The drawing under review shows one solid part. Ordinate dimensions are in mm from its lowest x, y, z. Give positions to 0.01 mm unless a question says otherwise; leave off trailing zeros. Order: outer loops, then holes, each group sorted by start corner. A loop starts at its lowest first (then second) coordinate and runs counter-clockwise, first axis right, second up. Notation, with made-up numbers: (27.25, -36) - (66.25, -36) arc R16 ccw to (66.25, -30) - close; hole circle Ø2 at (42.25, -2). An arc over 180 degrees is marked (long way). Use CSV: the item, a comma, the result in double quotes. Start each with the question number.
1. To check wall thickness, follow line 1 (Y direction, x = 57.15, z = 5); line 2 (Y direction, x = 58, z = 7.75); line 3 (X direction, y = 9.75, z = 4.5). State the ranges of each line that lie inside material, in increasing order. Write a range as [from, to].
2. Take a section at D-D, the plane y = 14. State the section outline as (x, z) points.
3. Draft analysis for pull direction X (two halves, no side actions). For the marked faces 1, 2, 3 and 4, state which applies: released by +X, released by -X, zero draft, split by the parting line, or undercut.
4. Take a section at B-B, the plane y = 11. State the section outline as (x, z) points (1 decimal), then the cut area to 3 significant figures.
5. Take a section at C-C, the plane z = 6. Count the separate pieces of the cut face and the enclosed holes in it, then the cut area to 3 significant figures.
6. Take a section at A-A, the plane x = 57.15. State the section outline as (y, z) points.
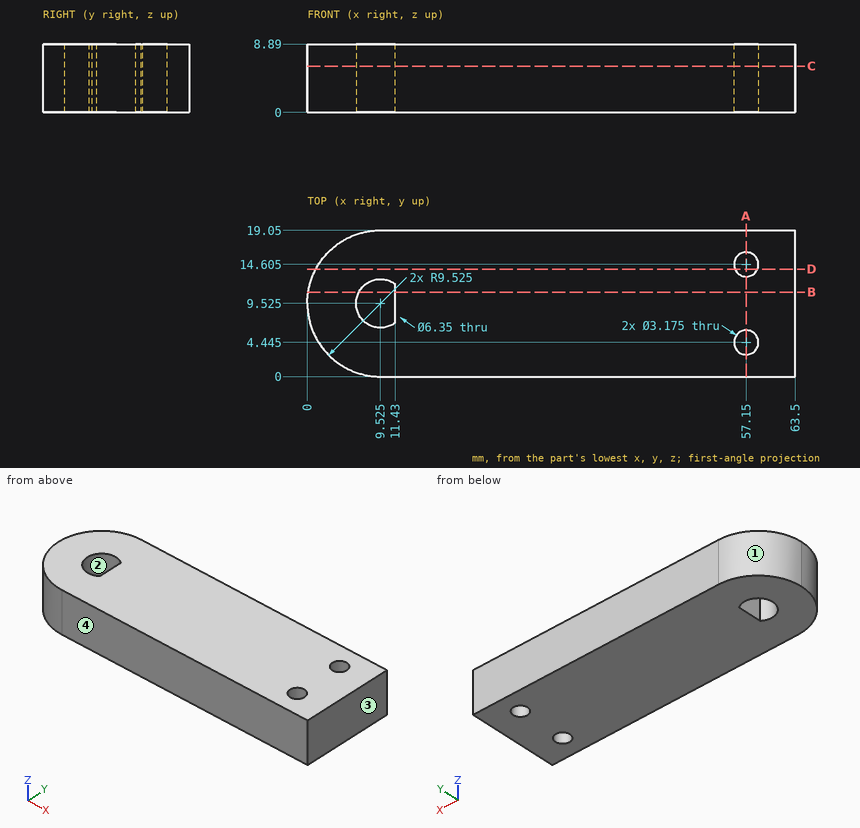
Determined:
1,line 1,"y = [0, 2.86], [6.03, 13.02], [16.19, 19.05]"
1,line 2,"y = [0, 3.1], [5.79, 13.26], [15.95, 19.05]"
1,line 3,"x = [0, 6.36], [11.43, 63.5]"
2,outline,"(1.12, 0) - (55.68, 0) - (55.68, 8.89) - (1.12, 8.89) - close; (58.62, 0) - (63.5, 0) - (63.5, 8.89) - (58.62, 8.89) - close"
3,face 1,"released by -X"
3,face 2,"undercut"
3,face 3,"released by +X"
3,face 4,"zero draft"
4,outline,"(0.1, 0) - (6.7, 0) - (6.7, 8.9) - (0.1, 8.9) - close; (11.4, 0) - (63.5, 0) - (63.5, 8.9) - (11.4, 8.9) - close"
4,area,"522 mm²"
5,separate pieces,"1"
5,enclosed holes,"3"
5,area,"1,130 mm²"
6,outline,"(0, 0) - (2.86, 0) - (2.86, 8.89) - (0, 8.89) - close; (6.03, 0) - (13.02, 0) - (13.02, 8.89) - (6.03, 8.89) - close; (16.19, 0) - (19.05, 0) - (19.05, 8.89) - (16.19, 8.89) - close"
